```python
from build123d import *

# Parameters (mm, degrees)
ESQUISSE1_R             = 11
BOSS_EXTRU_1_DEPTH      = 26
BOSS_EXTRU_2_DEPTH      = 1.5
ENL_V_MAT_EXTRU_1_DEPTH = 1.5
ESQUISSE4_R             = 3
BOSS_EXTRU_3_DEPTH      = 18


with BuildPart() as part:
    # Esquisse1 → Boss.-Extru.1 (new body)
    with BuildSketch(Plane.XY):
        with Locations(Location((0, 0, 0), (0, 0, 180))):
            Circle(ESQUISSE1_R)
    extrude(amount=BOSS_EXTRU_1_DEPTH)

    # Esquisse2 → Boss.-Extru.2 (add)
    with BuildSketch(Plane(origin=(0, 0, 0), x_dir=(-1, 0, 0), z_dir=(0, 0, -1))):
        with BuildLine():
            Line((-7.8, 11.625833303), (-19, 7.54936668))
            Line((-19, 7.54936668), (-19, 0))
            Line((-19, 0), (19, 0))
            Line((19, 0), (19, 7.54936668))
            Line((19, 7.54936668), (7.8, 11.625833303))
            ThreePointArc((7.8, 11.625833303), (0, 14), (-7.8, 11.625833303))
        make_face()
    boss_extru_2 = extrude(amount=BOSS_EXTRU_2_DEPTH)

    # Symétrie1: Boss.-Extru.2 across plane
    add(boss_extru_2.mirror(Plane(origin=(19, 0, -1.5), x_dir=(0, 0, 1), z_dir=(0, 1, 0))))

    # Esquisse3 → Enlèv. mat.-Extru.1 (cut)
    with BuildSketch(Plane(origin=(0, 0, -1.5), x_dir=(-1, 0, 0), z_dir=(0, 0, -1))):
        with BuildLine():
            ThreePointArc((-15.644312892, 3.907824988), (-16.124554191, 0), (-15.644312892, -3.907824988))
            ThreePointArc((-15.644312892, -3.907824988), (-13.825754742, -5), (-12.73357973, -3.181441851))
            ThreePointArc((-12.73357973, -3.181441851), (-13.124554191, 0), (-12.73357973, 3.181441851))
            ThreePointArc((-12.73357973, 3.181441851), (-13.825754742, 5), (-15.644312892, 3.907824988))
        make_face()
        with BuildLine():
            ThreePointArc((15.644132561, 3.908546838), (16.125446605, 0), (15.644132561, -3.908546838))
            ThreePointArc((15.644132561, -3.908546838), (13.825032892, -4.99981967), (12.733760061, -3.18072))
            ThreePointArc((12.733760061, -3.18072), (13.125446605, 0), (12.733760061, 3.18072))
            ThreePointArc((12.733760061, 3.18072), (13.825032892, 4.99981967), (15.644132561, 3.908546838))
        make_face()
    extrude(amount=-ENL_V_MAT_EXTRU_1_DEPTH, mode=Mode.SUBTRACT)

    # Esquisse4 → Boss.-Extru.3 (add)
    with BuildSketch(Plane(origin=(0, 0, -1.5), x_dir=(-1, 0, 0), z_dir=(0, 0, -1))):
        Circle(ESQUISSE4_R)
    extrude(amount=BOSS_EXTRU_3_DEPTH)


solid = part.part
```
Geometry check sheet. Reference: the model listing, model coordinates, mm. A direction names the side the tool comes from. Round coordinates to 2 decimals unless told otherwise and drop trailing zeros. Loops run counter-clockwise (first coordinate to the right, second up) from the corner with the lowest first, then second, coordinate; pieces in that order, holes last. Notation, with made-up numbers: M 2.5,-32 L 51.5,-32 A16 cw 51.5,-15 Z; hole C 45,2.5 d11. An arc over 180 degrees is marked long. Return JSON: item names as keys, results as strings. Group by question number.
(1) Section check B-B, the plane x = 0. Enter the section's corners in (y, z).
(2) Section check C-C, the plane z = -14.5. Enter the section's corners in (x, y).
(3) Go/stop test with flat-tipped pins: pin 1 (5 mm diameter, centred on y = 8, z = 5, fed in from +X); pin 2 (8 mm diameter, centred on x = -6, y = -5.5, fed in from -Z); pin 3 (3 mm diameter, centred on y = 0.5, z = 15.5, fed in from +X). Record where each tip stops, or that it passes through.
(4) Mould release check, pull along Y, two halves, no side actions. Record for faces 1 (the face through (-16.125, 0.055, -0.76)), 2 (the face through (13.322, 9.616, -0.74)), 3 (the face through (-19, 0, -1)): pulls with the +Y half, pulls with the -Y half, needs draft (parallel to the pull), parting line crosses it, or undercut.
(5) Section check A-A, the plane y = 0. Enter the section's corners in (x, z).
(6) Scan lines: line 1 along Z through (x, y) = (-10.5, 5.5); line 2 along Z through (x, y) = (6, 3); line 3 along Y through (x, z) = (0, 3). Record each from-to range of solid material in increasing order. Write a range as [from, to].
(7) Section check D-D, the plane y = -5.75. Enter the section's corners in (x, z), and give its area (3 significant figures).
(8) Set-up check for faces 4 (the face through (3, 0, -10)), 5 (the face through (16.124, 0.055, -0.76)), 6 (the face through (0, -14, -1)), 7 (the face through (-12, 0, 0)): record each of +Z, -Z, +X, -X, +Y, -Y from which the full face is reachable in a straight line by a thin tool's end or side.
Data:
{
 "1": {"outline": "M -14,-1.5 L -3,-1.5 L -3,-19.5 L 3,-19.5 L 3,-1.5 L 14,-1.5 L 14,0 L 11,0 L 11,26 L -11,26 L -11,0 L -14,0 Z"},
 "2": {"outline": "C 0,0 d6"},
 "3": {"pin 1": "x = 9.53", "pin 2": "z = -1.5", "pin 3": "x = 11"},
 "4": {"face 1": "undercut", "face 2": "pulls with the +Y half", "face 3": "needs draft"},
 "5": {"outline": "M -19,-1.5 L -16.13,-1.5 L -16.13,0 L -19,0 Z; M -13.13,-1.5 L -3,-1.5 L -3,-19.5 L 3,-19.5 L 3,-1.5 L 13.12,-1.5 L 13.12,0 L 11,0 L 11,26 L -11,26 L -11,0 L -13.13,0 Z; M 16.12,-1.5 L 19,-1.5 L 19,0 L 16.12,0 Z"},
 "6": {"line 1": "[-1.5, 0]", "line 2": "[-1.5, 26]", "line 3": "[-11, 11]"},
 "7": {"outline": "M -19,-1.5 L 19,-1.5 L 19,0 L 9.38,0 L 9.38,26 L -9.38,26 L -9.38,0 L -19,0 Z", "area": "545 mm²"},
 "8": {"face 4": "-Z", "face 5": "+Z, -Z", "face 6": "+Z, -Z, -Y", "face 7": "+Z"}
}
